```python
from build123d import *

# Parameters (mm, degrees)
EXTRUDE_2_DEPTH          = 16
SKETCH_3_R               = 1.65
CUT_EXTRUDE_1_DEPTH      = 126
CUT_EXTRUDE_1_DEPTH_BACK = 6
EXTRUDE_3_DEPTH          = 3
MIRROR_2_COPY_1_DEPTH    = 3


with BuildPart() as part:
    # 草图1 → 凸台-拉伸2 (new body)
    with BuildSketch(Plane.XY):
        Polygon((-65, 0), (65, 0), (65, -12), (60, -12), (60, -5), (-60, -5), (-60, -12), (-65, -12), align=None)
    extrude(amount=EXTRUDE_2_DEPTH)

    # 草图3 → 切除-拉伸1 (cut, two sides)
    with BuildSketch(Plane(origin=(-60, 0, 0), x_dir=(0, 0, -1), z_dir=(1, 0, 0))) as cut_extrude_1_sk:
        with Locations((-8, -9)):
            Circle(SKETCH_3_R)
    extrude(amount=CUT_EXTRUDE_1_DEPTH, mode=Mode.SUBTRACT)
    extrude(cut_extrude_1_sk.sketch, amount=-CUT_EXTRUDE_1_DEPTH_BACK, mode=Mode.SUBTRACT)

    # 草图4 → 凸台-拉伸3 (add)
    with BuildSketch(Plane(origin=(0, 0, 0), x_dir=(-1, 0, 0), z_dir=(0, 0, -1))):
        Polygon((54, -5), (60, -12), (60, -5), align=None)
    extrude_3 = extrude(amount=-EXTRUDE_3_DEPTH)

    # 镜向1: 凸台-拉伸3 across plane
    add(extrude_3.mirror(Plane.XY.offset(8)))

    # 镜向2: 凸台-拉伸3 across plane
    add(extrude_3.mirror(Plane(origin=(0, 0, 0), x_dir=(0, 0, 1), z_dir=(1, 0, 0))))

    # 镜向2 copy 1 sketch → 镜向2 copy 1 (add)
    with BuildSketch(Plane.XY.offset(16)):
        Polygon((54, -5), (60, -12), (60, -5), align=None)
    extrude(amount=-MIRROR_2_COPY_1_DEPTH)


solid = part.part
```
For this review, take the finished solid that the model builds, in its own axes (mm). A direction names the side the tool comes from. Round coordinates to 2 decimals unless told otherwise and drop trailing zeros. Loops run counter-clockwise (first coordinate to the right, second up) from the corner with the lowest first, then second, coordinate; pieces in that order, holes last.
Q1. To check wall thickness, follow line 1 along X through (y, z) = (-5.75, 3.5); line 2 along Y through (x, z) = (-63.6, 8); line 3 along Y through (x, z) = (4.5, 9.75). State the ranges of each line that lie inside material, in increasing order.
Result sheet:
line 1: x = -65 to -60, 60 to 65
line 2: y = -12 to -10.65, -7.35 to 0
line 3: y = -5 to 0
Q2. Add section D-D on x = -56.5. Write out the cut boundary in (y, z).
Result sheet:
outline: (-7.92, 0) - (0, 0) - (0, 16) - (-7.92, 16) - (-7.92, 13) - (-5, 13) - (-5, 3) - (-7.92, 3) - close
Q3. Insertion check: pin 1 Ø2 at (x, z) = (-12.5, 7) entering from -Y; pin 2 Ø2.5 at (y, z) = (-9, 8) entering from -X. Each pin has a flat end and moves straight along its axis. Give the tip position at first contact, or say it passes through.
Result sheet:
pin 1: stops at y = -5
pin 2: passes through
Q4. Add section B-B on y = -9. Write out the cut boundary in (x, z), plus the area to 3 significant figures.
Result sheet:
outline: (-65, 0) - (-57.43, 0) - (-57.43, 3) - (-60, 3) - (-60, 6.35) - (-65, 6.35) - close; (-65, 9.65) - (-60, 9.65) - (-60, 13) - (-57.43, 13) - (-57.43, 16) - (-65, 16) - close; (57.43, 0) - (65, 0) - (65, 6.35) - (60, 6.35) - (60, 3) - (57.43, 3) - close; (57.43, 13) - (60, 13) - (60, 9.65) - (65, 9.65) - (65, 16) - (57.43, 16) - close
area: 158 mm2
Q5. Machinability: for faces 1 (the face through (-57, -8.5, 1.5)), 2 (the face through (-58, -7, 3)), 3 (the face through (-1, 0, 8)), which of the approach directions +Z, -Z, +X, -X, +Y, -Y give a long, thin tool a straight path to every point of the face, cutting with its end or side? Answer none if there is none.
Result sheet:
face 1: +Z, -Z, -Y
face 2: -Y
face 3: +Z, -Z, +X, -X, +Y
Q6. Mouldability with a two-part tool opening along X and no side actions: class faces 4 (the face through (65, -6, 8)), 5 (the face through (63, -12, 8)), 6 (the face through (1, -5, 8)) as +X half, -X half, draft (parallel to the pull), parting line (faces both ways), or undercut.
Result sheet:
face 4: +X half
face 5: draft
face 6: undercut
Q7. Add section C-C on x = 17.5. Write out the cut boundary in (y, z).
Result sheet:
outline: (-5, 0) - (0, 0) - (0, 16) - (-5, 16) - close
Q8. Add section A-A on z = 8. Write out the cut boundary in (x, y), plus the area to 3 significant figures.
Result sheet:
outline: (-65, -12) - (-60, -12) - (-60, -10.65) - (-65, -10.65) - close; (-65, -7.35) - (-60, -7.35) - (-60, -5) - (60, -5) - (60, -7.35) - (65, -7.35) - (65, 0) - (-65, 0) - close; (60, -12) - (65, -12) - (65, -10.65) - (60, -10.65) - close
area: 687 mm2
